Could you check a few things on this model? Use its own coordinates, in mm. Face numbers are marked on the shaded views. A direction names the side the tool comes from. Give positions to 0.01 mm unless a question says otherwise; leave off trailing zeros. Loops run counter-clockwise (first coordinate to the right, second up) from the corner with the lowest first, then second, coordinate; pieces in that order, holes last. Notation, with made-up numbers: (51, 86) - (110, 86) arc R31 cw to (110, 115) - close; hole circle Ø7 at (33.25, 30.25). An arc over 180 degrees is marked (long way). Write each question's results on one line, items separated by ' | '. Start each with the question number.
1) I want a section at B-B, the plane y = 37. Write out the boundary of the cut face in (x, z) (3 decimals), and give its area (3 significant figures).
2) I want a section at C-C, the plane z = 0. Write out the boundary of the cut face in (x, y).
3) I'm going to push flat-ended pins straight in: pin 1 (12 mm diameter, centred on y = 60, z = 0, fed in from -X); pin 2 (0.6 mm diameter, centred on y = 102.5, z = 45, fed in from +X); pin 3 (5 mm diameter, centred on x = 14, y = 156, fed in from +Z) (3 decimals). Where does each tip first touch, or does it pass through?
4) On a 3-axis mill with a long thin cutter (end or side, diameter ignored), from which of +Z, -Z, +X, -X, +Y, -Y can I reach the whole of each face in a straight line? I mean the marked faces 4 and 5. Say none if no direction works.
5) I want a section at D-D, the plane x = -108.5. Write out the boundary of the cut face in (y, z) (3 decimals).
6) If we mould it in two halves opening along Y, with no side actions, what happens to the marked faces 1, 2 and 3? For each: +Y half, -Y half, draft (parallel to the pull), parting line (faces both ways), or undercut.
7) If I drill on probe 1 along X at (y, z) = (189, 32); probe 2 along Y at (x, z) = (-40, 32.5); probe 3 along Z at (x, y) = (-66.5, 10) (3 decimals), over which ranges is the centre line in solid material (lowest first)? Write a range as [from, to].
8) I want a section at A-A, the plane x = 30.5. Write out the boundary of the cut face in (y, z) (3 decimals).
from build123d import *

# Parameters (mm, degrees)
SKETCH2_W            = 203.2
SKETCH2_H            = 92.71
BOSS_EXTRUDE1_DEPTH  = 206.502
SKETCH3_W            = 190.5
SKETCH3_H            = 193.802
CUT_EXTRUDE1_DEPTH   = 86.36
CUT_EXTRUDE2_REACH   = 236.765
SKETCH6_W            = 264.16
SKETCH6_H            = 181.102
BOSS_EXTRUDE2_DEPTH  = 3.175
SKETCH8_W            = 4.064
SKETCH8_H            = 25.4
SKETCH8_W_2          = 6.35
SKETCH8_H_2          = 1.27
CUT_EXTRUDE3_DEPTH   = 31.75
FILLET1_R            = 1.27
BOSS_EXTRUDE3_DEPTH  = 12.7
FILLET1_OF_MIRROR1_R = 1.27


with BuildPart() as part:
    # Sketch2 → Boss-Extrude1 (new body)
    with BuildSketch(Plane(origin=(0, 0, 0), x_dir=(1, 0, 0), z_dir=(0, 1, 0))):
        Rectangle(SKETCH2_W, SKETCH2_H)
    extrude(amount=BOSS_EXTRUDE1_DEPTH)

    # Sketch3 → Cut-Extrude1 (cut)
    with BuildSketch(Plane.XY.offset(46.355)):
        with Locations((0, 103.251)):
            Rectangle(SKETCH3_W, SKETCH3_H)
    extrude(amount=-CUT_EXTRUDE1_DEPTH, mode=Mode.SUBTRACT)

    # Sketch5 → Cut-Extrude2 (cut, up to next)
    with BuildSketch(Plane.XZ.offset(-206.502), mode=Mode.PRIVATE) as cut_extrude2_sk1:
        with BuildLine():
            Line((-47.625, 31.115), (47.625, 31.115))
            ThreePointArc((47.625, 31.115), (78.74, 0), (47.625, -31.115))
            Line((47.625, -31.115), (-47.625, -31.115))
            ThreePointArc((-47.625, -31.115), (-78.74, 0), (-47.625, 31.115))
        make_face()
    cut_extrude2_tool1 = extrude(cut_extrude2_sk1.sketch, amount=CUT_EXTRUDE2_REACH, mode=Mode.PRIVATE) & part.part
    add(cut_extrude2_tool1.solids().sort_by_distance((0, 206.502, 0))[0], mode=Mode.SUBTRACT)

    # Sketch6 → Boss-Extrude2 (add)
    with BuildSketch(Plane(origin=(0, 0, -46.355), x_dir=(-1, 0, 0), z_dir=(0, 0, -1))):
        with Locations((0, 90.551)):
            Rectangle(SKETCH6_W, SKETCH6_H)
    extrude(amount=BOSS_EXTRUDE2_DEPTH)

    # Sketch8 → Cut-Extrude3 (cut)
    with BuildSketch(Plane.XY.offset(46.355)):
        with Locations((-97.282, 115.951)):
            Rectangle(SKETCH8_W, SKETCH8_H)
        Polygon((-95.25, 103.251), (-99.314, 103.251), (-101.6, 103.251), (-101.6, 101.981), (-95.25, 101.981), align=None)
        with Locations((-98.425, 129.286)):
            Rectangle(SKETCH8_W_2, SKETCH8_H_2)
    cut_extrude3 = extrude(amount=-CUT_EXTRUDE3_DEPTH, mode=Mode.SUBTRACT)

    # Fillet1
    fillet1_edges = [part.edges().sort_by_distance(p)[0] for p in [
        (-99.314, 115.951, 14.605),
    ]]
    fillet(fillet1_edges, radius=FILLET1_R)

    # Sketch10 → Boss-Extrude3 (add, symmetric)
    with BuildSketch(Plane(origin=(0, 103.251, 0), x_dir=(-1, 0, 0), z_dir=(0, -1, 0))):
        Polygon((101.6, -46.355), (102.807721606, -45.657721606), (102.807721606, -44.387721606), (101.6, -43.18), align=None)
    boss_extrude3 = extrude(amount=BOSS_EXTRUDE3_DEPTH, both=True)

    # Mirror1: Cut-Extrude3, Boss-Extrude3 across plane
    add(cut_extrude3.mirror(Plane(origin=(0, 0, 0), x_dir=(0, 0, 1), z_dir=(1, 0, 0))), mode=Mode.SUBTRACT)
    add(boss_extrude3.mirror(Plane(origin=(0, 0, 0), x_dir=(0, 0, 1), z_dir=(1, 0, 0))))

    # Fillet1 of Mirror1
    fillet1_of_mirror1_edges = [part.edges().sort_by_distance(p)[0] for p in [
        (99.314, 115.951, 14.605),
    ]]
    fillet(fillet1_of_mirror1_edges, radius=FILLET1_OF_MIRROR1_R)


solid = part.part
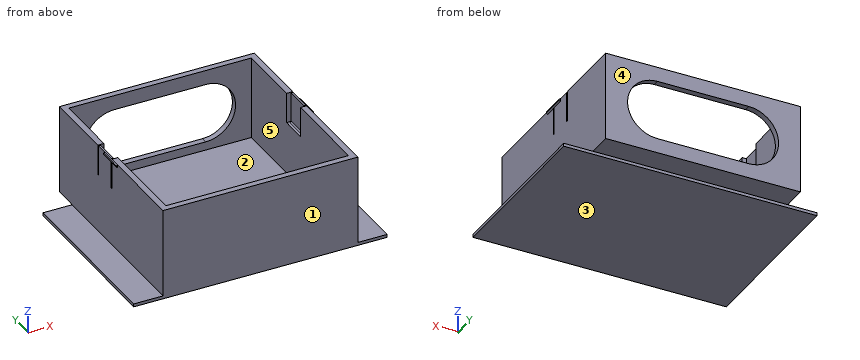
Answers:
1) outline: (-132.08, -49.53) - (132.08, -49.53) - (132.08, -46.355) - (101.6, -46.355) - (101.6, 46.355) - (95.25, 46.355) - (95.25, -40.005) - (-95.25, -40.005) - (-95.25, 46.355) - (-101.6, 46.355) - (-101.6, -46.355) - (-132.08, -46.355) - close | area: 3,230 mm2
2) outline: (-101.6, 0) - (101.6, 0) - (101.6, 206.5) - (78.74, 206.5) - (78.74, 200.15) - (95.25, 200.15) - (95.25, 6.35) - (-95.25, 6.35) - (-95.25, 200.15) - (-78.74, 200.15) - (-78.74, 206.5) - (-101.6, 206.5) - close
3) pin 1: stops at x = -101.6 | pin 2: stops at x = 102.81 | pin 3: stops at z = -40.005
4) face 4: +Z, -Z, +X, -X, +Y | face 5: +Z
5) outline: (0, -49.53) - (181.102, -49.53) - (181.102, -46.355) - (0, -46.355) - close
6) face 1: -Y half | face 2: undercut | face 3: draft
7) probe 1: x = [-101.6, -95.25], [95.25, 101.6] | probe 2: y = [0, 6.35], [200.15, 206.5] | probe 3: z = [-49.53, -40.005]
8) outline: (0, -49.53) - (181.102, -49.53) - (181.102, -46.355) - (206.502, -46.355) - (206.502, -31.115) - (200.152, -31.115) - (200.152, -40.005) - (6.35, -40.005) - (6.35, 46.355) - (0, 46.355) - close; (200.152, 31.115) - (206.502, 31.115) - (206.502, 46.355) - (200.152, 46.355) - close
